Autodesk Fusion 360 part; units mm, degrees
sketch "Sketch1" plane through (0, 0, 0) normal (0, 0, 1) x (1, 0, 0)
  line L0 (0, 0) -> (214, 0)
  line L1 (214, 0) -> (214, 10)
  line L2 (214, 10) -> (0, 10)
  line L3 (0, 10) -> (0, 0)
extrude "Extrude1" add sketch "Sketch1" along normal blind 12 makes body 1
sketch "Sketch2" plane through (0, 0, 0) normal (0, 0, 1) x (1, 0, 0)
  line L0 (-5, 2) -> (0, 2)
  line L1 (0, 2) -> (0, 8)
  line L2 (0, 8) -> (-5, 8)
  line L3 (-5, 8) -> (-5, 2)
extrude "Extrude2" add sketch "Sketch2" along normal blind 6 from surface at 3 separate body makes body 2
sketch "Sketch3" plane through (0, 0, 0) normal (0, 0, 1) x (1, 0, 0)
  line L0 (214, 2) -> (219, 2)
  line L1 (219, 2) -> (219, 8)
  line L2 (219, 8) -> (214, 8)
  line L3 (214, 8) -> (214, 2)
extrude "Extrude3" add sketch "Sketch3" along normal blind 6 from surface at 3 separate body makes body 3
combine "Combine1" operation add target body 1 tool bodies 2 3
Could you check a few things on this model? Use its own coordinates, in mm. A direction names the side the tool comes from. Round coordinates to 2 decimals unless told otherwise and drop trailing zeros. Write each loop counter-clockwise with the first axis right and the second up, starting at its lowest first coordinate (ties: lowest second). Pieces come first, ordered by that corner, then holes. Notation, with made-up numbers: M 0,19 L 53,19 A15 cw 53,40 Z; hole C -13.75,49.25 d11. An arc over 180 degrees is marked long. Answer in a Markdown table with one row per item. Add a question column.
Q1. Imagine slicing it at A-A (z = 6.75). Please give me the cut outline in (x, y), then the cut area to 3 significant figures.
Q2. Will these pins go through, and if not, where does the flat tip stop? pin 1 Ø2.5 at (x, y) = (-2.5, 4) entering from -Z; pin 2 Ø1.5 at (x, z) = (216.5, 5) entering from +Y; pin 3 Ø1.5 at (x, z) = (-2.5, 7) entering from -Y.
Q3. On a 3-axis mill with a long thin cutter (end or side, diameter ignored), from which of +Z, -Z, +X, -X, +Y, -Y can I reach the whole of each face in a straight line? I mean faces 1 (the flat face through (-3, 5, 9)), 2 (the flat face through (-2, 8, 6)), 3 (the flat face through (216, 5, 9)). Say none if no direction works.
Q4. Imagine slicing it at B-B (y = 4.25). Please give me the cut outline in (x, z), then the cut area to 3 significant figures.
Q5. If I drill on line 1 (X direction, y = 1, z = 3.5), over which ranges is the centre line in solid material (lowest first)? Write a range as from..to.
Values:
| question | item | result |
|---|---|---|
| 1 | outline | M -5,2 L 0,2 L 0,0 L 214,0 L 214,2 L 219,2 L 219,8 L 214,8 L 214,10 L 0,10 L 0,8 L -5,8 Z |
| 1 | area | 2,200 mm^2 |
| 2 | pin 1 | z = 3 |
| 2 | pin 2 | y = 8 |
| 2 | pin 3 | y = 2 |
| 3 | face 1 | +Z, -X, +Y, -Y |
| 3 | face 2 | +Z, -Z, -X, +Y |
| 3 | face 3 | +Z, +X, +Y, -Y |
| 4 | outline | M -5,3 L 0,3 L 0,0 L 214,0 L 214,3 L 219,3 L 219,9 L 214,9 L 214,12 L 0,12 L 0,9 L -5,9 Z |
| 4 | area | 2,630 mm^2 |
| 5 | line 1 | 0..214 |
